Source: CAD feature listing. Evaluate the final solid. Frame: model axes, mm. A direction names the side the tool comes from. Round coordinates to 2 decimals unless told otherwise and drop trailing zeros. Loops run counter-clockwise (first coordinate to the right, second up) from the corner with the lowest first, then second, coordinate; pieces in that order, holes last. Notation, with made-up numbers: M 43,39.25 L 93,39.25 A19 cw 93,72.25 Z; hole C 5.5,67.25 d10. An arc over 180 degrees is marked long. Answer as a JSON object with one key per item and string values.
from build123d import *

# Parameters (mm, degrees)
F0_R      = 12.7
F1_DEPTH  = 50.8
F2_W      = 56.316178
F2_H      = 24.083158
F3_DEPTH  = 25.4
F5_DEPTH  = 34.544
F8_DEPTH  = 25.4
F7_R      = 4.89521
F9_DEPTH  = 127
F6_R      = 5.04868
F10_DEPTH = 25.4


with BuildPart() as f1:
    # F0 (on Top) → F1 (new body)
    with BuildSketch(Plane.XY):
        with BuildLine():
            Line((68.180415, 25.4), (-58.776217, 25.4))
            ThreePointArc((-58.776217, 25.4), (-84.176217, 0), (-58.776217, -25.4))
            Line((-58.776217, -25.4), (68.180415, -25.4))
            ThreePointArc((68.180415, -25.4), (93.580415, 0), (68.180415, 25.4))
        make_face()
        with Locations((-58.776217, 0)):
            Circle(F0_R, mode=Mode.SUBTRACT)
        with Locations((68.180415, 0)):
            Circle(F0_R, mode=Mode.SUBTRACT)
    extrude(amount=F1_DEPTH)

    # F2 (on face) → F3 (join)
    with BuildSketch(Plane.XY.offset(50.8)):
        Rectangle(F2_W, F2_H)
    extrude(amount=F3_DEPTH)

    # F4 (on face) → F5 (cut)
    with BuildSketch(Plane.XZ.offset(12.041579)):
        with BuildLine():
            Line((-7.62, 76.2), (-7.62, 60.96))
            ThreePointArc((-7.62, 60.96), (0, 53.34), (7.62, 60.96))
            Line((7.62, 60.96), (7.62, 76.2))
            Line((7.62, 76.2), (-7.62, 76.2))
        make_face()
    extrude(amount=-F5_DEPTH, mode=Mode.SUBTRACT)

    # F7 (on face) → F8 (cut)
    with BuildSketch(Plane.YZ.offset(28.158089)):
        with BuildLine():
            ThreePointArc((-12.041579, 66.644274), (0.202546, 75.187594), (12.041579, 66.09121))
            Line((12.041579, 66.09121), (12.041579, 76.2))
            Line((12.041579, 76.2), (-12.041579, 76.2))
            Line((-12.041579, 76.2), (-12.041579, 66.644274))
        make_face()
    extrude(amount=-F8_DEPTH, mode=Mode.SUBTRACT)

    # F7 (on face) → F9 (cut)
    with BuildSketch(Plane.YZ.offset(28.158089)):
        with Locations((-0.087499, 62.557597)):
            Circle(F7_R)
    extrude(amount=-F9_DEPTH, mode=Mode.SUBTRACT)

    # F6 (on face) → F10 (cut)
    with BuildSketch(Plane(origin=(-28.158089, 0, 0), x_dir=(0, -1, 0), z_dir=(-1, 0, 0))):
        with BuildLine():
            ThreePointArc((-12.041579, 66.459917), (0.065622, 74.940473), (12.041579, 66.275567))
            Line((12.041579, 66.275567), (12.041579, 76.2))
            Line((12.041579, 76.2), (-12.041579, 76.2))
            Line((-12.041579, 76.2), (-12.041579, 66.459917))
        make_face()
        with Locations((-0.031925, 62.197081)):
            Circle(F6_R)
    extrude(amount=-F10_DEPTH, mode=Mode.SUBTRACT)


solid = f1.part
Item 1: Section A-A on z = 31.5. Return the cut outline in (x, y).
Answer sheet:
{"outline": "M -58.78,-25.4 L 68.18,-25.4 A25.4 ccw 68.18,25.4 L -58.78,25.4 A25.4 ccw Z; hole C -58.78,0 d25.4; hole C 68.18,0 d25.4"}
Item 2: Access query for faces 1 (the flat face through (-28.158, -3, 57)), 2 (the cylindrical face through (-17.75, -1.55, 67.23)), 3 (the flat face through (0, -12.042, 53)). Directions: +Z, -Z, +X, -X, +Y, -Y. A direction counts if a zero-diameter tool reaches every point of the face in a straight line with its end or side. Return the directions, or none.
Answer sheet:
{"face 1": "+Z, -X, +Y, -Y", "face 2": "+X, -X", "face 3": "+Z, +X, -X, -Y"}
Item 3: Section C-C on y = 9. Return the cut outline in (x, z), then the cut area to 3 significant figures.
Answer sheet:
{"outline": "M -82.53,0 L -67.74,0 L -67.74,50.8 L -82.53,50.8 Z; M -49.82,0 L 59.22,0 L 59.22,50.8 L 28.16,50.8 L 28.16,71.33 L 7.62,71.33 L 7.62,60.96 A7.62 cw -7.62,60.96 L -7.62,71.25 L -28.16,71.25 L -28.16,50.8 L -49.82,50.8 Z; M 77.14,0 L 91.93,0 L 91.93,50.8 L 77.14,50.8 Z", "area": "7,950 mm²"}
Item 4: Pull-direction query (Y, two-part tool) for faces 4 (the flat face through (3, 0, 0)), 5 (the cylindrical face through (-46.66, 3.81, 25.04)), 6 (the cylindrical face through (93.574, -0.559, 25.044)), 7 (the cylindrical face through (-17.53, 1.75, 57.45)); classes: pulls with the +Y half, pulls with the -Y half, needs draft (parallel to the pull), parting line crosses it, or undercut.
Answer sheet:
{"face 4": "needs draft", "face 5": "undercut", "face 6": "parting line crosses it", "face 7": "undercut"}
Item 5: Contact query for flat-ended pins moving along their axis: pin 1 Ø5 at (x, y) = (-64.5, -17.5) entering from +Z; pin 2 Ø11 at (y, z) = (1.5, 67) entering from +X; pin 3 Ø10 at (y, z) = (7.5, 48.5) entering from +X. Output: stop coordinate, or through.
Answer sheet:
{"pin 1": "stops at z = 50.8", "pin 2": "stops at x = 28.16", "pin 3": "stops at x = 93.46"}
Item 6: Section D-D on x = 0. Return the cut outline in (y, z), then the cut area to 3 significant figures.
Answer sheet:
{"outline": "M -25.4,0 L 25.4,0 L 25.4,50.8 L 12.04,50.8 L 12.04,53.34 L -12.04,53.34 L -12.04,50.8 L -25.4,50.8 Z", "area": "2,640 mm²"}
Item 7: Section B-B on y = 0. Return the cut outline in (x, z), then the cut area to 3 significant figures.
Answer sheet:
{"outline": "M -84.18,0 L -71.48,0 L -71.48,50.8 L -84.18,50.8 Z; M -46.08,0 L 55.48,0 L 55.48,50.8 L 28.16,50.8 L 28.16,57.66 L 6.87,57.66 A7.62 cw -6.6,57.15 L -28.16,57.15 L -28.16,50.8 L -46.08,50.8 Z; M -28.16,67.45 L -7.62,67.45 L -7.62,74.94 L -28.16,74.94 Z; M 7.62,67.45 L 28.16,67.45 L 28.16,75.19 L 7.62,75.19 Z; M 80.88,0 L 93.58,0 L 93.58,50.8 L 80.88,50.8 Z", "area": "7,100 mm²"}
Item 8: Line query: probe 1 along X at (y, z) = (7, 66.5); probe 2 along Z at (x, y) = (51, -18); probe 3 along Y at (x, z) = (76, 11.5). Output: solid intervals per line, ascending. Write a range as from..to.
Answer sheet:
{"probe 1": "x = -28.16..-7.62, 7.62..28.16", "probe 2": "z = 0..50.8", "probe 3": "y = -24.17..-10.01, 10.01..24.17"}
